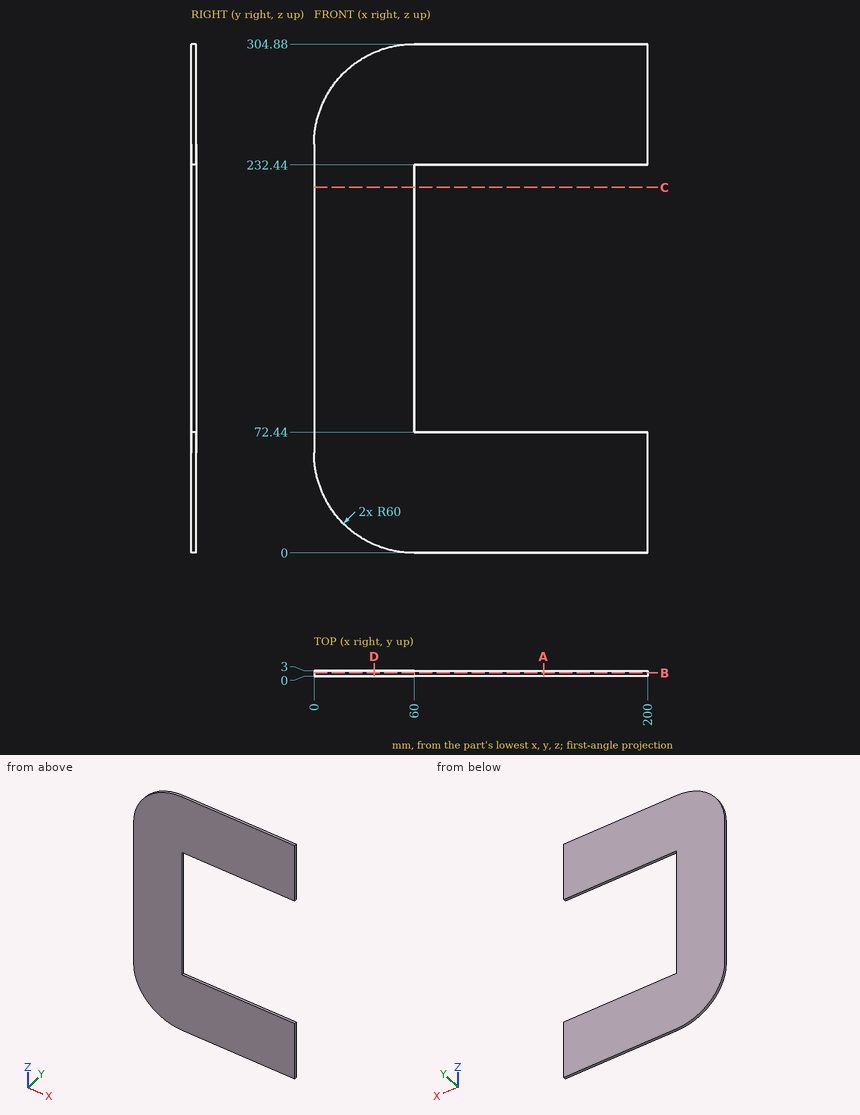
The drawing under review shows one solid part. Ordinate dimensions are in mm from its lowest x, y, z. Give positions to 0.01 mm unless a question says otherwise; leave off trailing zeros. Write each loop counter-clockwise with the first axis right and the second up, starting at its lowest first coordinate (ties: lowest second). Pieces come first, ordered by that corner, then holes.
1. Add section A-A, the plane x = 137.5. Write out the cut boundary in (y, z).
2. Add section D-D, the plane x = 36. Write out the cut boundary in (y, z), plus the area to 3 significant figures.
3. For P1, Ø1, axis at y = 2.5, z = 221, coming from the -X side, flat-tipped, find the tip position at first contact; note if it passes through.
4. Add section B-B, the plane y = 1.9. Write out the cut boundary in (x, z).
5. Add section C-C, the plane z = 219. Write out the cut boundary in (x, y).
6. Wall thickness on L1, parallel to Z at x = 189, y = 2.3; L2, parallel to X at y = 1.05, z = 154.5; L3, parallel to X at y = 1, z = 292.5: over which ranges is each line inside the solid? List them lowest first.
Worked answers:
1. outline: (0, 0) - (3, 0) - (3, 72.44) - (0, 72.44) - close; (0, 232.44) - (3, 232.44) - (3, 304.88) - (0, 304.88) - close
2. outline: (0, 5.01) - (3, 5.01) - (3, 299.87) - (0, 299.87) - close
2. area: 885 mm2
3. P1: stops at x = 0
4. outline: (0, 60) arc R60 ccw to (60, 0) - (200, 0) - (200, 72.44) - (60, 72.44) - (60, 232.44) - (200, 232.44) - (200, 304.88) - (60, 304.88) arc R60 ccw to (0, 244.88) - close
5. outline: (0, 0) - (60, 0) - (60, 3) - (0, 3) - close
6. L1: z = 0 to 72.44, 232.44 to 304.88
6. L2: x = 0 to 60
6. L3: x = 23.5 to 200
